Geometry: see drawing. Coordinates: mm, zero at the bounding-box minimum. A direction names the side the tool comes from. Coordinates: 2 decimals unless noted, no trailing zeros. Write each loop counter-clockwise with the first axis right and the second up, starting at its lowest first coordinate (ties: lowest second). Pieces come first, ordered by that corner, then holes.
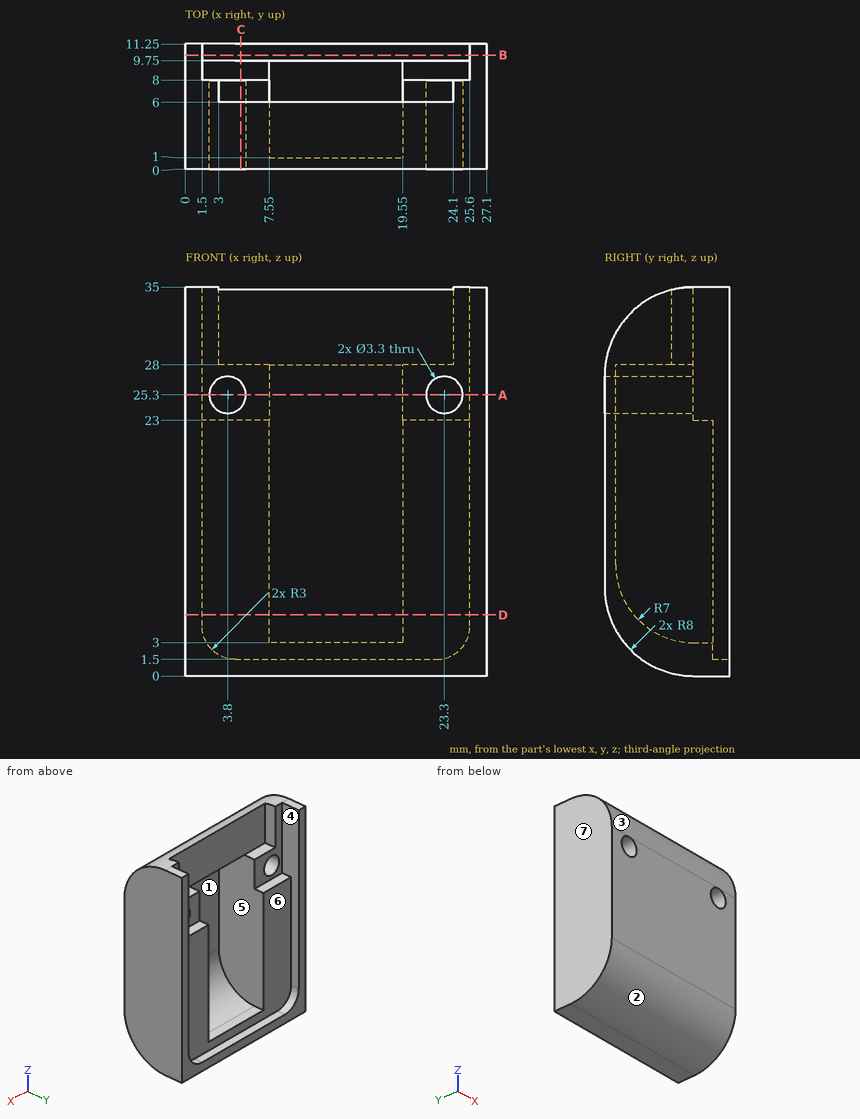
Item 1: Section B-B, the plane y = 10.25. Output: boundary loops of the cut face in (x, z).
Derived:
outline: (0, 0) - (27.1, 0) - (27.1, 35) - (25.6, 35) - (25.6, 4.5) arc R3 cw to (22.6, 1.5) - (4.5, 1.5) arc R3 cw to (1.5, 4.5) - (1.5, 35) - (0, 35) - close
Item 2: Set-up query: the marked faces 5, 6 and 7. Return all of +Z, -Z, +X, -X, +Y, -Y with unobstructed straight access to the full face (end or side cutting, diameter ignored); none if empty.
Derived:
face 5: +Y
face 6: +Z, +Y
face 7: +Z, -Z, -X, +Y, -Y
Item 3: Material intervals for probe 1 along X at (y, z) = (2.5, 16); probe 2 along X at (y, z) = (8.25, 30); probe 3 along X at (y, z) = (4, 25), sorted ascending.
Derived:
probe 1: x = 0 to 7.55, 19.55 to 27.1
probe 2: x = 0 to 1.5, 25.6 to 27.1
probe 3: x = 0 to 2.18, 5.42 to 7.55, 19.55 to 21.68, 24.92 to 27.1
Item 4: Section D-D, the plane z = 5.5. Output: boundary loops of the cut face in (x, y).
Derived:
outline: (0, 0.4) - (27.1, 0.4) - (27.1, 11.25) - (25.6, 11.25) - (25.6, 9.75) - (19.55, 9.75) - (19.55, 2.64) - (7.55, 2.64) - (7.55, 9.75) - (1.5, 9.75) - (1.5, 11.25) - (0, 11.25) - close
Item 5: Section C-C, the plane x = 5. Output: boundary loops of the cut face in (y, z).
Derived:
outline: (0, 8) arc R8 ccw to (8, 0) - (11.25, 0) - (11.25, 1.5) - (9.75, 1.5) - (9.75, 23) - (8, 23) - (8, 24.17) - (0, 24.17) - close; (0, 26.43) - (8, 26.43) - (8, 28) - (6, 28) - (6, 34.75) arc R8 ccw to (0, 27) - close
Item 6: Pin query (flat end, axial travel): pin 1 (1 mm diameter, centred on x = 19.5, z = 23, fed in from +Y); pin 2 (4.5 mm diameter, centred on x = 23.3, z = 25.3, fed in from +Y); pin 3 (6 mm diameter, centred on x = 11.5, z = 23, fed in from +Y). Return the tip coordinate at first contact, or that it passes through.
Derived:
pin 1: stops at y = 9.75
pin 2: stops at y = 8
pin 3: stops at y = 1
Item 7: Pull-direction query (Z, two-part tool) for the marked faces 1, 2, 3 and 4; classes: released by +Z, released by -Z, zero draft, split by the parting line, or undercut.
Derived:
face 1: undercut
face 2: released by -Z
face 3: released by +Z
face 4: zero draft
Item 8: Section A-A, the plane z = 25.3. Output: boundary loops of the cut face in (x, y).
Derived:
outline: (0, 0) - (2.15, 0) - (2.15, 8) - (1.5, 8) - (1.5, 11.25) - (0, 11.25) - close; (5.45, 0) - (21.65, 0) - (21.65, 8) - (19.55, 8) - (19.55, 1) - (7.55, 1) - (7.55, 8) - (5.45, 8) - close; (24.95, 0) - (27.1, 0) - (27.1, 11.25) - (25.6, 11.25) - (25.6, 8) - (24.95, 8) - close
